```python
from build123d import *

# Parameters (mm, degrees)
ESQUISSE1_W             = 40
ESQUISSE1_H             = 18
BOSS_EXTRU_1_DEPTH      = 12
ESQUISSE2_W             = 40
ESQUISSE2_H             = 12
BOSS_EXTRU_2_DEPTH      = 10
ENL_V_MAT_EXTRU_1_DEPTH = 12
ESQUISSE4_R             = 2.5
ENL_V_MAT_EXTRU_2_DEPTH = 28
ESQUISSE5_R             = 2.5
ENL_V_MAT_EXTRU_3_DEPTH = 12
ESQUISSE6_R             = 4
ENL_V_MAT_EXTRU_5_DEPTH = 12
ESQUISSE7_W             = 12
ESQUISSE7_H             = 18
BOSS_EXTRU_3_DEPTH      = 15
ESQUISSE8_W             = 12
ESQUISSE8_H             = 18
BOSS_EXTRU_4_DEPTH      = 15
ESQUISSE9_R             = 2.5
ENL_V_MAT_EXTRU_6_DEPTH = 12
CONG_1_R                = 2


with BuildPart() as part:
    # Esquisse1 → Boss.-Extru.1 (new body)
    with BuildSketch(Plane.XY):
        with Locations((3.185612757, 0.725848564)):
            Rectangle(ESQUISSE1_W, ESQUISSE1_H)
    extrude(amount=BOSS_EXTRU_1_DEPTH)

    # Esquisse2 → Boss.-Extru.2 (add)
    with BuildSketch(Plane.XZ.offset(8.274151436)):
        with Locations((3.185612757, 6)):
            Rectangle(ESQUISSE2_W, ESQUISSE2_H)
    extrude(amount=BOSS_EXTRU_2_DEPTH)

    # Esquisse3 → Enlèv. mat.-Extru.1 (cut)
    with BuildSketch(Plane.XY.offset(12)):
        with BuildLine():
            Line((-2.864387243, -18.274151436), (9.235612757, -18.274151436))
            ThreePointArc((9.235612757, -18.274151436), (3.185612757, -12.224151436), (-2.864387243, -18.274151436))
        make_face()
    extrude(amount=-ENL_V_MAT_EXTRU_1_DEPTH, mode=Mode.SUBTRACT)

    # Esquisse4 → Enlèv. mat.-Extru.2 (cut)
    with BuildSketch(Plane.XZ.offset(18.274151436)):
        with Locations(Location((-9.839387243, 6, 0), (0, 0, 270))):
            Circle(ESQUISSE4_R)
        with Locations(Location((16.210612757, 6, 0), (0, 0, 270))):
            Circle(ESQUISSE4_R)
    extrude(amount=-ENL_V_MAT_EXTRU_2_DEPTH, mode=Mode.SUBTRACT)

    # Esquisse5 → Enlèv. mat.-Extru.3 (cut)
    with BuildSketch(Plane.XY.offset(12)):
        with Locations((3.185612757, 0.725848564)):
            Circle(ESQUISSE5_R)
    extrude(amount=-ENL_V_MAT_EXTRU_3_DEPTH, mode=Mode.SUBTRACT)

    # Esquisse6 → Enlèv. mat.-Extru.5 (cut)
    with BuildSketch(Plane(origin=(0, 9.725848564, 0), x_dir=(1, 0, 0), z_dir=(0, 1, 0))):
        with Locations(Location((16.210612757, -6, 0), (0, 0, 270))):
            Circle(ESQUISSE6_R)
        with Locations(Location((-9.839387243, -6, 0), (0, 0, 270))):
            Circle(ESQUISSE6_R)
    extrude(amount=-ENL_V_MAT_EXTRU_5_DEPTH, mode=Mode.SUBTRACT)

    # Esquisse7 → Boss.-Extru.3 (add)
    with BuildSketch(Plane.ZY.offset(16.814387243)):
        with Locations((6, 0.725848564)):
            Rectangle(ESQUISSE7_W, ESQUISSE7_H)
    extrude(amount=BOSS_EXTRU_3_DEPTH)

    # Esquisse8 → Boss.-Extru.4 (add)
    with BuildSketch(Plane(origin=(23.185612757, 0, 0), x_dir=(0, 0, -1), z_dir=(1, 0, 0))):
        with Locations((-6, 0.725848564)):
            Rectangle(ESQUISSE8_W, ESQUISSE8_H)
    extrude(amount=BOSS_EXTRU_4_DEPTH)

    # Esquisse9 → Enlèv. mat.-Extru.6 (cut)
    with BuildSketch(Plane.XY.offset(12)):
        with Locations((-24.314387243, 0.725848564)):
            Circle(ESQUISSE9_R)
        with Locations((30.685612757, 0.725848564)):
            Circle(ESQUISSE9_R)
    extrude(amount=-ENL_V_MAT_EXTRU_6_DEPTH, mode=Mode.SUBTRACT)

    # Congé1
    cong_1_edges = [part.edges().sort_by_distance(p)[0] for p in [
        (3.185612757, 9.725848564, 0),
        (23.185612757, -13.274151436, 0),
        (-16.814387243, -13.274151436, 0),
        (-16.814387243, -8.274151436, 6),
        (-24.314387243, -8.274151436, 0),
        (-31.814387243, 0.725848564, 0),
        (-31.814387243, -8.274151436, 6),
        (-31.814387243, 9.725848564, 6),
        (30.685612757, -8.274151436, 0),
        (23.185612757, -8.274151436, 6),
        (38.185612757, 0.725848564, 0),
        (38.185612757, 9.725848564, 6),
        (38.185612757, -8.274151436, 6),
    ]]
    fillet(cong_1_edges, radius=CONG_1_R - 0.0001)  # a hair under: the kernel refuses the full size


solid = part.part
```
Part model, mm, in its own coordinate system. A direction names the side the tool comes from. Round coordinates to 2 decimals unless told otherwise and drop trailing zeros. Order: outer loops, then holes, each group sorted by start corner. A loop starts at its lowest first (then second) coordinate and runs counter-clockwise, first axis right, second up. Notation, with made-up numbers: M -27.5,-10.5 L -12.5,-10.5 A23 ccw -12.5,12.5 Z; hole C 42,88 d7. An arc over 180 degrees is marked long. Answer in a Markdown table with one row per item. Add a question column.
Q1. Cut at D-D on z = 6.75. Give the number of separate pieces and of enclosed holes in the cut face, and give its area (3 significant figures).
Q2. Cut at B-B on y = -3.75. Give the cut face in (x, z).
Q3. Mould opens along Z. For faces 1 (the face through (20.177, 3.81, 5.479)), 2 (the face through (23.186, -14, 7)), 3 (the face through (30.8, -7.7, 0.6)), 4 (the face through (3, -4, 12)) say: +Z half, -Z half, draft (parallel to the pull), parting line (faces both ways), or undercut.
Q4. Cut at C-C on z = 1. Give the cut face in (x, y).
Q5. 3-axis set-ups, long thin cutter, end or side, ignore diameter. For faces 5 (the face through (-24, -8.274, 7)), 6 (the face through (-16.24, -14.33, 0.6)), 7 (the face through (22.615, -14.33, 0.601)): which of +Z, -Z, +X, -X, +Y, -Y reach the whole face in a straight line?
Q6. Cut at A-A on x = 5. Give the cut face in (y, z), and give its area (3 significant figures).
Q7. Wall check: L1, parallel to X at y = -11.25, z = 6; L2, parallel to X at y = -5.75, z = 6; L3, parallel to X at y = -1.5, z = 0.5. Give the ranges that are in metal, low to high. Write a range as from..to.
Q8. Pin check, flat tips, straight feed: pin 1 (1 mm diameter, centred on y = -13.5, z = 5.5, fed in from -X); pin 2 (6 mm diameter, centred on x = -9.84, z = 6, fed in from +Y); pin 3 (2.5 mm diameter, centred on y = -14.5, z = 5, fed in from +X). Stop position of each tip, or through.
Established:
| question | item | result |
|---|---|---|
| 1 | separate pieces | 3 |
| 1 | enclosed holes | 3 |
| 1 | area | 1,200 mm2 |
| 2 | outline | M -31.81,2 A2 ccw -29.81,0 L 36.19,0 A2 ccw 38.19,2 L 38.19,12 L -31.81,12 Z; hole C -9.84,6 d5; hole C 16.21,6 d5 |
| 3 | face 1 | undercut |
| 3 | face 2 | draft |
| 3 | face 3 | -Z half |
| 3 | face 4 | +Z half |
| 4 | outline | M -31.55,-6.27 A1.73 ccw -29.81,-8.01 L -18.81,-8.01 A2.27 cw -16.55,-10.27 L -16.55,-18.27 L -2.86,-18.27 A6.05 cw 9.24,-18.27 L 22.92,-18.27 L 22.92,-10.27 A2.27 cw 25.19,-8.01 L 36.19,-8.01 A1.73 ccw 37.92,-6.27 L 37.92,7.73 A1.73 ccw 36.19,9.46 L -29.81,9.46 A1.73 ccw -31.55,7.73 Z; hole C -24.31,0.73 d5; hole C 3.19,0.73 d5; hole C 30.69,0.73 d5 |
| 5 | face 5 | +Z, -Z, -X, -Y |
| 5 | face 6 | -Z, -X, -Y |
| 5 | face 7 | -Z, +X, -Y |
| 6 | outline | M -12.5,0 L -0.99,0 L -0.99,12 L -12.5,12 Z; M 2.45,0 L 7.73,0 A2 ccw 9.73,2 L 9.73,12 L 2.45,12 Z |
| 6 | area | 225 mm2 |
| 7 | L1 | x = -16.81..-12.34, -7.34..13.71, 18.71..23.19 |
| 7 | L2 | x = -31.81..-12.34, -7.34..13.71, 18.71..38.19 |
| 7 | L3 | x = -31.14..-25.45, -23.18..2.05, 4.32..29.55, 31.82..37.51 |
| 8 | pin 1 | stops at x = -16.81 |
| 8 | pin 2 | stops at y = -2.27 |
| 8 | pin 3 | stops at x = 23.19 |
